Here's how the part is built. I have some questions about the finished solid (model axes, mm). A direction names the side the tool comes from. Round coordinates to 2 decimals unless told otherwise and drop trailing zeros. Order: outer loops, then holes, each group sorted by start corner. A loop starts at its lowest first (then second) coordinate and runs counter-clockwise, first axis right, second up.
Autodesk Inventor part; units mm, degrees
ref_plane "YZ Plane" through (0, 0, 0) normal (1, 0, 0) x (0, 1, 0)
ref_plane "XZ Plane" through (0, 0, 0) normal (0, 1, 0) x (-1, 0, 0)
ref_plane "XY Plane" through (0, 0, 0) normal (0, 0, 1) x (1, 0, 0)
sketch "スケッチ1" plane through (0, 0, 0) normal (0, 1, 0) x (-1, 0, 0)
  line L0 (-7.5, -10) -> (7.5, -10)
  line L1 (7.5, -10) -> (7.5, 10)
  line L2 (7.5, 10) -> (-7.5, 10)
  line L3 (-7.5, 10) -> (-7.5, -10)
  line L4 (-7.5, -10) -> (7.5, 10) construction
  line L5 (7.5, -10) -> (-7.5, 10) construction
  line L6 (-7.5, 10) -> (7.5, 10)
  line L7 (7.5, 10) -> (7.5, 4)
  line L8 (7.5, 4) -> (-7.5, 4)
  line L9 (-7.5, 4) -> (-7.5, 10)
  line L10 (-7.5, -10) -> (7.5, -10)
  line L11 (7.5, -10) -> (7.5, -4)
  line L12 (7.5, -4) -> (-7.5, -4)
  line L13 (-7.5, -4) -> (-7.5, -10)
  point P0 (0, 0)
  dimension "d0" = 15
  dimension "d1" = 20
  dimension "d2" = 6
  dimension "d3" = 6
extrude "押し出し1" add sketch "スケッチ1" along normal blind 6 contours L3 L12 L1 L0 | L3 L2 L1 L8
sketch "スケッチ2" plane through (0, 6, 0) normal (0, 1, 0) x (1, 0, 0)
  line L0 (7.5, 10) -> (-7.5, 10)
  line L1 (-7.5, 10) -> (-7.5, 4)
  line L2 (-7.5, 4) -> (7.5, 4)
  line L3 (7.5, 4) -> (7.5, 10)
  line L4 (-7.5, -5.5) -> (7.5, -5.5)
  line L5 (7.5, -5.5) -> (7.5, 5.5)
  line L6 (7.5, 5.5) -> (-7.5, 5.5)
  line L7 (-7.5, 5.5) -> (-7.5, -5.5)
  line L8 (-7.5, -5.5) -> (7.5, 5.5) construction
  line L9 (7.5, -5.5) -> (-7.5, 5.5) construction
  point P0 (0, 0)
  dimension "d6" = 11
extrude "押し出し2" add sketch "スケッチ2" along normal blind 20 contours L3 L2 L1 L6 | L5 L4 L7 L2
sketch "スケッチ3" plane through (7.5, 0, -4) normal (1, 0, 0) x (0, 0, -1)
  line L0 (1.5, 6) -> (1.5, 26)
  line L1 (-9.5, 26) -> (1.5, 26)
  line L2 (-9.5, 26) -> (1.5, 25.0376)
  point P0 (-4, 0)
  dimension "d9" = 5
extrude "押し出し3" cut sketch "スケッチ3" against normal blind 20
sketch "スケッチ4" plane through (-7.5, 26, 5.5) normal (0, 0.9961947, -0.0871557) x (1, 0, 0)
  line L0 (0, 0) -> (0, 11.042)
  line L1 (0, 0) -> (15, 0)
  line L2 (15, 11.042) -> (15, 0)
  line L3 (0, 11.042) -> (15, 11.042)
  line L4 (-2, 13.042) -> (17, 13.042)
  line L5 (17, 13.042) -> (17, -2)
  line L6 (17, -2) -> (-2, -2)
  line L7 (-2, -2) -> (-2, 13.042)
  point P0 (7.5, 7.7451)
  dimension "d12" = 2
  dimension "d13" = 2
  dimension "d14" = 2
  dimension "d15" = 2
extrude "押し出し4" add sketch "スケッチ4" along normal blind 15 contours L0 L3 L2 L1 | L4 L5 L6 L7
sketch "スケッチ5" plane through (9.5, 24.8633, -7.4924) normal (0, -0.0871557, -0.9961947) x (-1, 0, 0)
  line L0 (19, 0) -> (0, 0)
  line L1 (11.6915, 7.5253) -> (11.6915, 2.7045)
  line L2 (11.6915, 2.7045) -> (7.6915, 2.7045)
  line L3 (7.6915, 2.7045) -> (7.6915, 7.5253)
  line L4 (9.6915, 7.5253) -> (11.6915, 2.7045) construction
  line L5 (9.6915, 7.5253) -> (7.6915, 2.7045) construction
  line L6 (7.6915, 7.5253) -> (11.6915, 7.5253)
  line L7 (11.6915, 5.1149) -> (13.1915, 5.1149)
  line L8 (13.1915, 5.1149) -> (13.1915, 1.1149)
  line L9 (13.1915, 1.1149) -> (11.6915, 1.1149)
  line L10 (11.6915, 1.1149) -> (11.6915, 5.1149)
  line L11 (7.6915, 5.1149) -> (6.1915, 5.1149)
  line L12 (6.1915, 5.1149) -> (6.1915, 1.1149)
  line L13 (6.1915, 1.1149) -> (7.6915, 1.1149)
  line L14 (7.6915, 1.1149) -> (7.6915, 5.1149)
  line L15 (11.6915, 7.5253) -> (14.6915, 7.5253)
  line L16 (14.6915, 7.5253) -> (14.6915, 10.5253)
  line L17 (14.6915, 10.5253) -> (11.6915, 10.5253)
  line L18 (11.6915, 10.5253) -> (11.6915, 7.5253)
  line L19 (7.6915, 7.5253) -> (4.6915, 7.5253)
  line L20 (4.6915, 7.5253) -> (4.6915, 10.5253)
  line L21 (4.6915, 10.5253) -> (7.6915, 10.5253)
  line L22 (7.6915, 10.5253) -> (7.6915, 7.5253)
  point P0 (9.5, -25.4217)
  dimension "d18" = 4
  dimension "d19" = 1.5
  dimension "d20" = 4
  dimension "d21" = 1.5
  dimension "d22" = 3
  dimension "d23" = 3
  dimension "d24" = 3
  dimension "d25" = 2.7045
extrude "押し出し5" cut sketch "スケッチ5" against normal blind 1
sketch "スケッチ6" plane through (7.5, 0, 10) normal (1, 0, 0) x (0, 0, -1)
  line L0 (4.5, 6) -> (4.5, 26)
  line L1 (0, 6) -> (4.5, 6)
  line L2 (0, 0) -> (0, 6)
  line L3 (0, 0) -> (6, 0)
  line L4 (6, 0) -> (6, 6)
  line L5 (6, 6) -> (14, 6)
  line L6 (14, 0) -> (14, 6)
  line L7 (14, 0) -> (20, 0)
  line L8 (20, 0) -> (20, 6)
  line L9 (15.5, 6) -> (20, 6)
  line L10 (15.5, 6) -> (15.5, 25.0376)
  line L11 (15.5, 25.0376) -> (4.5, 25.0376)
  point P0 (10, 0)
extrude "押し出し6" cut sketch "スケッチ6" against normal blind 100
sketch "スケッチ7" plane through (-7.5, 25.0376, 5.5) normal (-1, 0, 0) x (0, 0, 1)
  line L0 (-11, 0) -> (0, 0)
  line L1 (0, 0) -> (0, 0.9624)
  line L2 (0, 0.9624) -> (-11, 0)
  point P0 (-5.5, -25.0376)
extrude "押し出し7" cut sketch "スケッチ7" against normal blind 100
sketch "スケッチ8" plane through (9.5, 24.8633, -7.4924) normal (0, -0.0871557, -0.9961947) x (-1, 0, 0)
  line L0 (19, 0) -> (0, 0)
  line L1 (19, 0) -> (19, 15)
  line L2 (0, 15) -> (19, 15)
  line L3 (0, 0) -> (0, 15)
  line L4 (1, 15) -> (1, 0)
  line L5 (18, 15) -> (18, 0)
  point P0 (9.5, -25.4217)
  dimension "d32" = 1
  dimension "d33" = 1
extrude "押し出し8" cut sketch "スケッチ8" against normal blind 100 contours L0 L5 L2 L1 | L0 L3 L2 L4
1) I'm going to push flat-ended pins straight in: pin 1 (1 mm diameter, centred on x = 1.5, y = 34.5, fed in from -Z); pin 2 (5 mm diameter, centred on x = 2, y = 29, fed in from -Z); pin 3 (1 mm diameter, centred on x = -6, z = 1, fed in from +Y). Where does each tip first touch, or does it pass through?
2) If we section it at A-A (y = 30.5): Write out the boundary of the cut face in (x, z).
3) I need wall thicknesses on line 1 (Y direction, x = 3.25, z = -6); line 2 (Y direction, x = -3, z = -0.5); line 3 (Z direction, x = 3, y = 39). Which ranges of each line are inside material? Lowest first, please.
4) If we section it at D-D (y = 28): Write out the boundary of the cut face in (x, z).
5) If we section it at C-C (z = -6): Write out the boundary of the cut face in (x, y).
6) For faces 5 (the flat face through (2.55, 30, -7.45)), 6 (the flat face through (-0.22, 27.6, -7.24)), which set-ups out of +Z, -Z, +X, -X, +Y, -Y let a thin tool reach every point of the face, with its end or its side?
7) If we section it at B-B (x = -4.75): Write out the boundary of the cut face in (y, z).
8) We'd pull the mould along Y, two halves only. Please class faces 1 (the flat face through (-8.5, 33, -1)), 2 (the flat face through (0.119, 33.541, 6.848)), 3 (the flat face through (-0.119, 33.89, -8.282)), 4 (the flat face through (-2.192, 34, -8)): +Y half, -Y half, draft (parallel to the pull), parting line (faces both ways), or undercut.
Solutions:
1. pin 1: stops at z = -8.38
1. pin 2: stops at z = -8.07
1. pin 3: stops at y = 40.71
2. outline: (-8.5, -7.99) - (-2.19, -7.99) - (-2.19, -6.98) - (1.81, -6.98) - (1.81, -7.99) - (8.5, -7.99) - (8.5, 7.11) - (-8.5, 7.11) - close
3. line 1: y = 24.99 to 40.05
3. line 2: y = 25.48 to 40.53
3. line 3: z = -8.73 to 6.37
4. outline: (-8.5, -7.77) - (-3.69, -7.77) - (-3.69, -6.76) - (3.31, -6.76) - (3.31, -7.77) - (8.5, -7.77) - (8.5, 7.33) - (-8.5, 7.33) - close
5. outline: (-8.5, 24.99) - (8.5, 24.99) - (8.5, 40.05) - (-8.5, 40.05) - close
6. face 5: none
6. face 6: -Z
7. outline: (24.86, -7.49) - (32.36, -8.15) - (32.45, -7.15) - (35.44, -7.41) - (35.35, -8.41) - (39.81, -8.8) - (41.12, 6.19) - (26.17, 7.49) - (26, 5.5) - (25.04, -5.5) - close
8. face 1: draft
8. face 2: +Y half
8. face 3: -Y half
8. face 4: undercut
